```python
from build123d import *

# Parameters (mm, degrees)
F0_W     = 60
F0_H     = 58
F1_DEPTH = 3
F4_DEPTH = 3
F6_DEPTH = 3


with BuildPart() as f1:
    # F0 (on Front) → F1 (new body)
    with BuildSketch(Plane.XZ):
        with Locations((0, -1)):
            Rectangle(F0_W, F0_H)
    extrude(amount=-F1_DEPTH)

    # F3 (on face) → F4 (join)
    with BuildSketch(Plane.XZ):
        Polygon((28, -28), (-28, -28), (-28, 28), (-30, 28), (-30, -30), (30, -30), (30, 28), (28, 28), align=None)
    extrude(amount=F4_DEPTH)

    # F5 (on face) → F6 (join)
    with BuildSketch(Plane.XZ.offset(3)):
        with BuildLine():
            Line((-30, 28), (-30, -30))
            Line((-30, -30), (30, -30))
            Line((30, -30), (30, 28))
            Line((30, 28), (28, 28))
            Line((28, 28), (27.9462553992, 3.5910797608))
            ThreePointArc((27.9462553992, 3.5910797608), (27.9999321267, 1.7954129877), (27.9383484068, 0))
            ThreePointArc((27.9383484068, 0), (0, -26.1429355685), (-27.9383484068, 0))
            ThreePointArc((-27.9383484068, 0), (-27.9999321267, 1.7954129877), (-27.9462553992, 3.5910797608))
            Line((-27.9462553992, 3.5910797608), (-28, 28))
            Line((-28, 28), (-30, 28))
        make_face()
        with BuildLine():
            Line((-27.9383484068, 0), (-27.9462553992, 3.5910797608))
            ThreePointArc((-27.9462553992, 3.5910797608), (-27.9999321267, 1.7954129877), (-27.9383484068, 0))
        make_face()
        with BuildLine():
            ThreePointArc((27.9383484068, 0), (27.9999321267, 1.7954129877), (27.9462553992, 3.5910797608))
            Line((27.9462553992, 3.5910797608), (27.9383484068, 0))
        make_face()
    extrude(amount=F6_DEPTH)


solid = f1.part
```
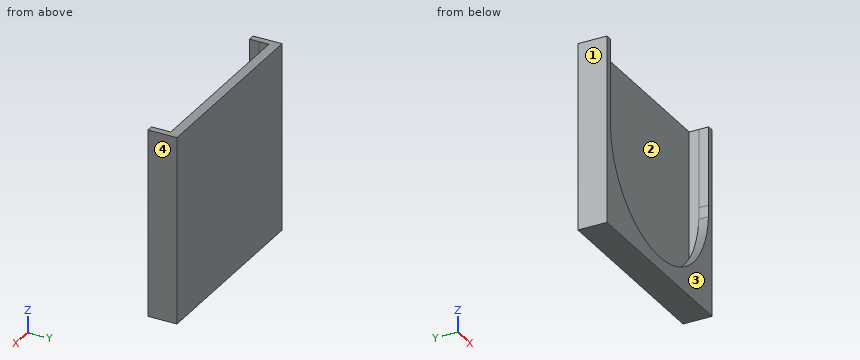
Build history of the part. All positions in model axes, mm. Face numbers are marked on the shaded views. Coordinates: 2 decimals unless noted, no trailing zeros. Order: outer loops, then holes, each group sorted by start corner. A loop starts at its lowest first (then second) coordinate and runs counter-clockwise, first axis right, second up.
Item 1: Saw through at A-A on y = -1.5. List the corners of the cut face in (x, z).
Filled in:
outline: (-30, -30) - (30, -30) - (30, 28) - (28, 28) - (28, -28) - (-28, -28) - (-28, 28) - (-30, 28) - close
Item 2: Drop flat-ended pins along their axis: pin 1 Ø3.5 at (x, y) = (-13, -1) entering from +Z; pin 2 Ø1.5 at (x, z) = (1.5, -15) entering from -Y. Give the stop position or say it passes through.
Filled in:
pin 1: stops at z = 28
pin 2: stops at y = 0
Item 3: Drill centre lines: L1, parallel to Y at x = -11.5, z = -24; L2, parallel to X at y = -1.75, z = -17.5; L3, parallel to Y at x = -26.5, z = 8.5. Where is each one in solid material? Low to high.
Filled in:
L1: y = -6 to -3, 0 to 3
L2: x = -30 to -28, 28 to 30
L3: y = 0 to 3
Item 4: Saw through at D-D on z = -15. List the corners of the cut face in (x, y).
Filled in:
outline: (-30, -6) - (-22.36, -6) - (-22.36, -3) - (-28, -3) - (-28, 0) - (28, 0) - (28, -3) - (22.36, -3) - (22.36, -6) - (30, -6) - (30, 3) - (-30, 3) - close
Item 5: Saw through at B-B on x = 0. List the corners of the cut face in (y, z), then the cut area to 3 significant figures.
Filled in:
outline: (-6, -30) - (3, -30) - (3, 28) - (0, 28) - (0, -28) - (-3, -28) - (-3, -26.14) - (-6, -26.14) - close
area: 192 mm2
Item 6: Mould opens along X. For the marked faces 1, 2, 3 and 4 say: released by +X, released by -X, zero draft, split by the parting line, or undercut.
Filled in:
face 1: released by -X
face 2: undercut
face 3: zero draft
face 4: released by +X
